Geometry check sheet. Reference: drawing and pictorial views, mm from the part's lowest x, y, z. Give positions to 0.01 mm unless a question says otherwise; leave off trailing zeros. Loops run counter-clockwise (first coordinate to the right, second up) from the corner with the lowest first, then second, coordinate; pieces in that order, holes last. Notation, with made-up numbers: (58, -14.75) - (84, -14.75) arc R24 cw to (84, 17.25) - close; hole circle Ø7 at (53, 1). An arc over 180 degrees is marked (long way). Answer in a Markdown table with one row per item. Add a question column.
(1) Sectioned sample at B-B on x = 33. Enter the section's corners in (y, z).
(2) Draft check along X on the marked faces 1, 2 and 3. Enter one of: released by +X, released by -X, zero draft, split by the parting line, or undercut.
(3) Go/stop test with flat-tipped pins: P1, Ø3, axis at y = 14.5, z = 31.5, coming from the -X side; P2, Ø3, axis at y = 3, z = 24, coming from the +X side; P3, Ø1, axis at y = 10.5, z = 34.5, coming from the -X side. Record where each tip stops, or that it passes through.
(4) Sectioned sample at A-A on z = 20.32. Enter the section's corners in (x, y), then the cut area to 3 significant figures.
(5) Sectioned sample at C-C on y = 10. Enter the section's corners in (x, z).
(6) Thickness scan on L1, parallel to X at y = 15, z = 20.32; L2, parallel to Z at x = 19, y = 18.5; L3, parallel to Z at x = 25.5, y = 9.5. Record the ranges inside material, lowest first.
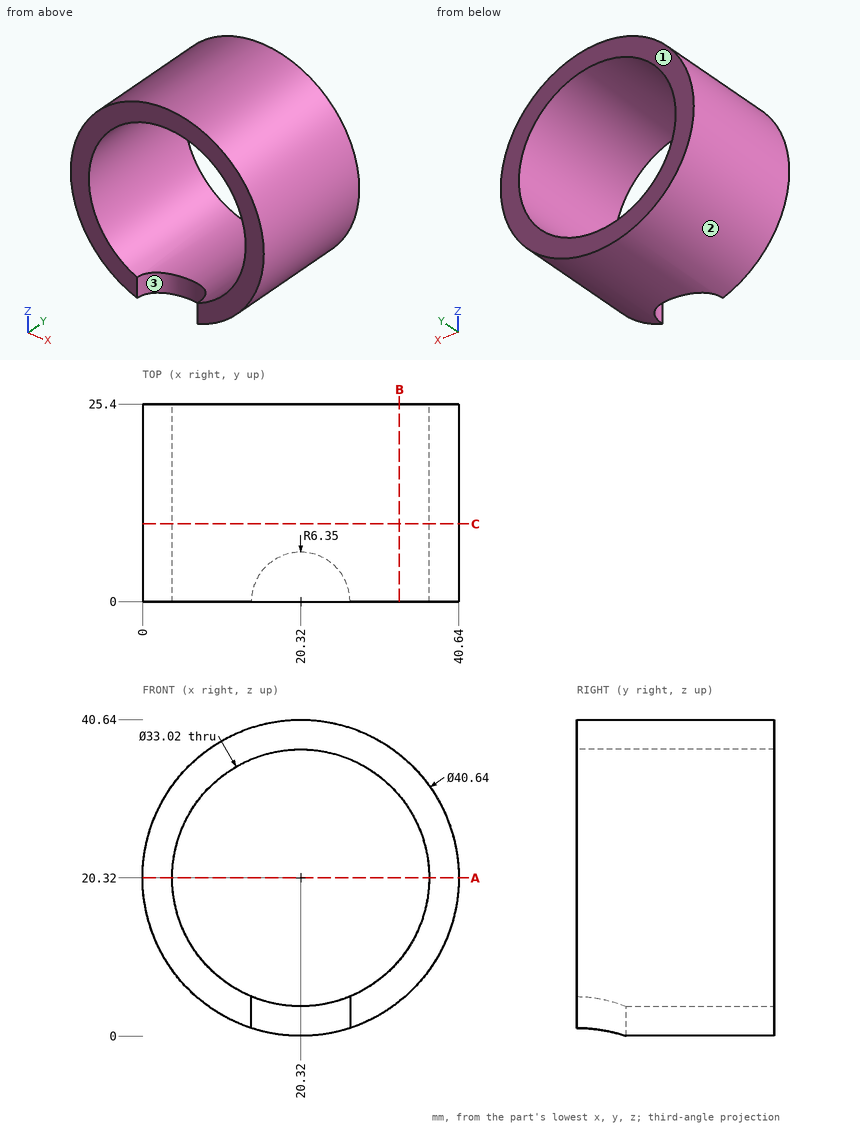
Reply:
| question | item | result |
|---|---|---|
| 1 | outline | (0, 4.44) - (25.4, 4.44) - (25.4, 9.75) - (0, 9.75) - close; (0, 30.89) - (25.4, 30.89) - (25.4, 36.2) - (0, 36.2) - close |
| 2 | face 1 | zero draft |
| 2 | face 2 | split by the parting line |
| 2 | face 3 | undercut |
| 3 | P1 | x = 2.45 |
| 3 | P2 | x = 40.52 |
| 3 | P3 | x = 5.29 |
| 4 | outline | (0, 0) - (3.81, 0) - (3.81, 25.4) - (0, 25.4) - close; (36.83, 0) - (40.64, 0) - (40.64, 25.4) - (36.83, 25.4) - close |
| 4 | area | 194 mm^2 |
| 5 | outline | circle Ø40.64 at (20.32, 20.32); hole circle Ø33.02 at (20.32, 20.32) |
| 6 | L1 | 0 to 3.81, 36.83 to 40.64 |
| 6 | L2 | 0.04 to 3.86, 36.78 to 40.6 |
| 6 | L3 | 0.67 to 4.64, 36 to 39.97 |
